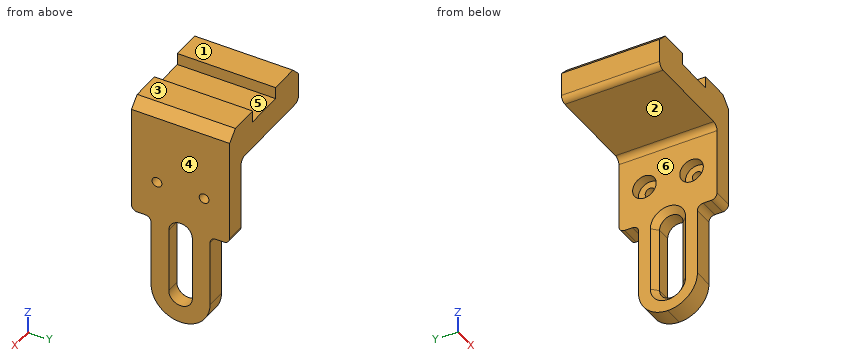
```python
from build123d import *

# Parameters (mm, degrees)
BOSS_EXTRUDE1_DEPTH = 25
SKETCH2_W           = 26
SKETCH2_H           = 5
CUT_EXTRUDE1_DEPTH  = 25
CUT_EXTRUDE2_DEPTH  = 25
FILLET1_R           = 1.5
SKETCH5_R           = 1.25
CUT_EXTRUDE4_DEPTH  = 25
CUT_EXTRUDE5_START  = -2.5
SKETCH5_4_R         = 3
SKETCH5_4_R_2       = 1.25
CUT_EXTRUDE5_DEPTH  = 2.5
SKETCH7_W           = 10
SKETCH7_H           = 3
CUT_EXTRUDE6_DEPTH  = 69.271516755
CHAMFER1_SIZE       = 2.5
FILLET2_R           = 1.5
CHAMFER2_SIZE       = 1.5


with BuildPart() as part:
    # Sketch1 → Boss-Extrude1 (new body)
    with BuildSketch(Plane(origin=(0, 0, 0), x_dir=(1, 0, 0), z_dir=(0, 1, 0))):
        Polygon((0, 0), (-30, 0), (-30, 10), (-5, 10), (-5, 56), (0, 56), align=None)
    extrude(amount=BOSS_EXTRUDE1_DEPTH)

    # Sketch2 → Cut-Extrude1 (cut)
    with BuildSketch(Plane(origin=(0, 0, 0), x_dir=(0, 0, -1), z_dir=(1, 0, 0))):
        with Locations((43, 22.5)):
            Rectangle(SKETCH2_W, SKETCH2_H)
        with BuildLine():
            Line((56, 12.5), (56, 20))
            Line((56, 20), (48.5, 20))
            ThreePointArc((48.5, 20), (53.803300859, 17.803300859), (56, 12.5))
        make_face()
        with BuildLine():
            Line((56, 5), (56, 12.5))
            ThreePointArc((56, 12.5), (53.803300859, 7.196699141), (48.5, 5))
            Line((48.5, 5), (56, 5))
        make_face()
        with Locations((43, 2.5)):
            Rectangle(SKETCH2_W, SKETCH2_H)
    extrude(amount=-CUT_EXTRUDE1_DEPTH, mode=Mode.SUBTRACT)

    # Sketch3 → Cut-Extrude2 (cut)
    with BuildSketch(Plane(origin=(0, 0, 0), x_dir=(0, 0, -1), z_dir=(1, 0, 0))):
        with BuildLine():
            Line((32, 15.5), (48.5, 15.5))
            ThreePointArc((48.5, 15.5), (51.5, 12.5), (48.5, 9.5))
            Line((48.5, 9.5), (32, 9.5))
            ThreePointArc((32, 9.5), (29, 12.5), (32, 15.5))
        make_face()
    extrude(amount=-CUT_EXTRUDE2_DEPTH, mode=Mode.SUBTRACT)

    # Fillet1
    fillet1_edges = [part.edges().sort_by_distance(p)[0] for p in [
        (-2.5, 25, -30),
        (-2.5, 20, -30),
        (-2.5, 0, -30),
        (-2.5, 5, -30),
    ]]
    fillet(fillet1_edges, radius=FILLET1_R)

    # Sketch5 → Cut-Extrude4 (cut)
    with BuildSketch(Plane(origin=(0, 0, 0), x_dir=(0, 0, -1), z_dir=(1, 0, 0))):
        with Locations((20, 18.5)):
            Circle(SKETCH5_R)
        with Locations((20, 6.5)):
            Circle(SKETCH5_R)
    extrude(amount=-CUT_EXTRUDE4_DEPTH, mode=Mode.SUBTRACT)

    # Sketch5_4 → Cut-Extrude5 (cut)
    # profile 1 of 2: a face of its own
    with BuildSketch(Plane(origin=(0, 0, 0), x_dir=(0, 0, -1), z_dir=(1, 0, 0)).offset(CUT_EXTRUDE5_START)):
        with Locations((20, 18.5)):
            Circle(SKETCH5_4_R)
        with Locations((20, 18.5)):
            Circle(SKETCH5_4_R_2, mode=Mode.SUBTRACT)
    # profile 2 of 2: a face of its own
    with BuildSketch(Plane(origin=(0, 0, 0), x_dir=(0, 0, -1), z_dir=(1, 0, 0)).offset(CUT_EXTRUDE5_START)):
        with Locations((20, 6.5)):
            Circle(SKETCH5_4_R)
        with Locations((20, 6.5)):
            Circle(SKETCH5_4_R_2, mode=Mode.SUBTRACT)
    extrude(amount=-CUT_EXTRUDE5_DEPTH, mode=Mode.SUBTRACT)

    # Sketch7 → Cut-Extrude6 (cut, through all)
    with BuildSketch(Plane(origin=(0, 25, 0), x_dir=(1, 0, 0), z_dir=(0, 1, 0))):
        with Locations((-15, 1.5)):
            Rectangle(SKETCH7_W, SKETCH7_H)
    extrude(amount=-CUT_EXTRUDE6_DEPTH, mode=Mode.SUBTRACT)

    # Chamfer1
    chamfer1_edges = [part.edges().sort_by_distance(p)[0] for p in [
        (0, 12.5, 0),
        (-30, 12.5, 0),
    ]]
    chamfer(chamfer1_edges, length=CHAMFER1_SIZE)

    # Fillet2
    fillet2_edges = [part.edges().sort_by_distance(p)[0] for p in [
        (-5, 12.5, -10),
        (-30, 12.5, -10),
    ]]
    fillet(fillet2_edges, radius=FILLET2_R)

    # Chamfer2
    chamfer2_edges = [part.edges().sort_by_distance(p)[0] for p in [
        (-5, 9.5, -40.25),
        (-5, 12.5, -51.5),
        (-5, 15.5, -40.25),
        (-5, 12.5, -29),
    ]]
    chamfer(chamfer2_edges, length=CHAMFER2_SIZE)


solid = part.part
```
Build history of the part. All positions in model axes, mm. Face numbers are marked on the shaded views. A direction names the side the tool comes from. Round coordinates to 2 decimals unless told otherwise and drop trailing zeros. Loops run counter-clockwise (first coordinate to the right, second up) from the corner with the lowest first, then second, coordinate; pieces in that order, holes last.
Item 1: Saw through at B-B (x = -4.25). List the corners of the cut face in (y, z).
Item 2: Saw through at D-D (z = -37.5). List the corners of the cut face in (x, y).
Item 3: Saw through at C-C (y = 6.5). List the corners of the cut face in (x, z), then the cut area to 4 significant figures.
Item 4: Pin check, flat tips, straight feed: P1, Ø1, axis at x = -2.5, y = 3, coming from the -Z side; P2, Ø1.5, axis at x = -20.5, y = 20.5, coming from the -Z side; P3, Ø2, axis at y = 18.5, z = -20, coming from the -X side; P4, Ø1, axis at y = 6.5, z = -28, coming from the -X side. Stop position of each tip, or through.
Item 5: Which spindle directions (+Z, -Z, +X, -X, +Y, -Y) get a long thin tool onto all of the face, cutting with end or side? Do the marked faces 1 and 2. Say none if no direction does.
Item 6: Two-plate mould, pull along X, no slides. Class the marked faces 3, 4, 5 and 6: released by +X, released by -X, zero draft, split by the parting line, or undercut.
Item 7: Saw through at A-A (z = -20). List the corners of the cut face in (x, y).
Item 8: Drill centre lines: line 1 along Y through (x, z) = (-1.1, -20); line 2 along X through (y, z) = (19.25, -31.5); line 3 along X through (y, z) = (12, -2.5). Where is each one in solid material? Low to high.
Worked answers:
1. outline: (0, -28.5) arc R1.5 ccw to (1.5, -30) - (3.5, -30) arc R1.5 cw to (5, -31.5) - (5, -48.5) arc R7.5 ccw to (20, -48.5) - (20, -31.5) arc R1.5 cw to (21.5, -30) - (23.5, -30) arc R1.5 ccw to (25, -28.5) - (25, 0) - (0, 0) - close; hole circle Ø6 at (6.5, -20); hole (8.75, -48.5) arc R3.75 ccw to (16.25, -48.5) - (16.25, -32) arc R3.75 ccw to (8.75, -32) - close; hole circle Ø6 at (18.5, -20)
2. outline: (-5, 5) - (0, 5) - (0, 9.5) - (-3.5, 9.5) - (-5, 8) - close; (-5, 17) - (-3.5, 15.5) - (0, 15.5) - (0, 20) - (-5, 20) - close
3. outline: (-30, -8.5) arc R1.5 ccw to (-28.5, -10) - (-6.5, -10) arc R1.5 cw to (-5, -11.5) - (-5, -17) - (-2.5, -17) - (-2.5, -18.75) - (0, -18.75) - (0, -2.5) - (-2.5, 0) - (-10, 0) - (-10, -3) - (-20, -3) - (-20, 0) - (-27.5, 0) - (-30, -2.5) - close; (-5, -53) - (0, -53) - (0, -21.25) - (-2.5, -21.25) - (-2.5, -23) - (-5, -23) - close
3. area: 457.5 mm2
4. P1: stops at z = -30
4. P2: stops at z = -10
4. P3: passes through
4. P4: stops at x = -5
5. face 1: +Z, +X, -X, +Y, -Y
5. face 2: -Z, -X, +Y, -Y
6. face 3: zero draft
6. face 4: released by +X
6. face 5: undercut
6. face 6: released by -X
7. outline: (-5, 0) - (0, 0) - (0, 5.25) - (-2.5, 5.25) - (-2.5, 3.5) - (-5, 3.5) - close; (-5, 9.5) - (-2.5, 9.5) - (-2.5, 7.75) - (0, 7.75) - (0, 17.25) - (-2.5, 17.25) - (-2.5, 15.5) - (-5, 15.5) - close; (-5, 21.5) - (-2.5, 21.5) - (-2.5, 19.75) - (0, 19.75) - (0, 25) - (-5, 25) - close
8. line 1: y = 0 to 5.25, 7.75 to 17.25, 19.75 to 25
8. line 2: x = -5 to 0
8. line 3: x = -30 to -20, -10 to 0
